Design review of the part built by this model. Coordinates are the model's own, in mm. Coordinates: 2 decimals unless noted, no trailing zeros. Loops run counter-clockwise (first coordinate to the right, second up) from the corner with the lowest first, then second, coordinate; pieces in that order, holes last. Notation, with made-up numbers: (16, 76.5) -> (37, 76.5) arc R17 cw to (37, 84.5) -> close; hole circle Ø5 at (47, -19.5). An arc over 180 degrees is marked (long way). Answer as a JSON object with one key per item and string values.
```python
from build123d import *

# Parameters (mm, degrees)
SKETCH1_W           = 698.5
SKETCH1_H           = 711.2
SKETCH1_W_2         = 203.2
SKETCH1_H_2         = 203.2
BOSS_EXTRUDE1_DEPTH = 1.5875
FILLET1_R           = 6.35
SKETCH2_R           = 2.667
SKETCH2_R_2         = 3.429
SKETCH2_R_3         = 3.175
SKETCH2_R_4         = 3.3782
SKETCH2_R_5         = 1.838164507
SKETCH2_R_6         = 1.838724473
CUT_EXTRUDE1_DEPTH  = 997.850144283
SKETCH3_W           = 50.8
SKETCH3_H           = 127
CUT_EXTRUDE2_DEPTH  = 997.850144283
SKETCH4_W           = 12.7
SKETCH4_H           = 50.8
CUT_EXTRUDE3_DEPTH  = 997.850144283
FILLET2_R           = 6.35


with BuildPart() as part:
    # Sketch1 → Boss-Extrude1 (new body)
    with BuildSketch(Plane(origin=(0, 0, 0), x_dir=(1, 0, 0), z_dir=(0, 1, 0))):
        with Locations((349.25, -355.6)):
            Rectangle(SKETCH1_W, SKETCH1_H)
        with Locations((133.35, -355.6)):
            Rectangle(SKETCH1_W_2, SKETCH1_H_2, mode=Mode.SUBTRACT)
        with Locations((565.15, -355.6)):
            Rectangle(SKETCH1_W_2, SKETCH1_H_2, mode=Mode.SUBTRACT)
    extrude(amount=BOSS_EXTRUDE1_DEPTH)

    # Fillet1
    fillet1_edges = [part.edges().sort_by_distance(p)[0] for p in [
        (31.75, 0.79375, 254),
        (31.75, 0.79375, 457.2),
        (234.95, 0.79375, 457.2),
        (234.95, 0.79375, 254),
        (463.55, 0.79375, 254),
        (463.55, 0.79375, 457.2),
        (666.75, 0.79375, 457.2),
        (666.75, 0.79375, 254),
    ]]
    fillet(fillet1_edges, radius=FILLET1_R)

    # Sketch2 → Cut-Extrude1 (cut, through all)
    with BuildSketch(Plane(origin=(0, 1.5875, 0), x_dir=(1, 0, 0), z_dir=(0, 1, 0))):
        with Locations(Location((440.3852, -407.797, 0), (0, 0, 270))):
            Circle(SKETCH2_R)
        with Locations(Location((258.1148, -407.797, 0), (0, 0, 270))):
            Circle(SKETCH2_R)
        with Locations(Location((258.1148, -303.403, 0), (0, 0, 270))):
            Circle(SKETCH2_R)
        with Locations(Location((440.3852, -303.403, 0), (0, 0, 270))):
            Circle(SKETCH2_R)
        with Locations(Location((460.248, -190.725477854, 0), (0, 0, 270))):
            Circle(SKETCH2_R_2)
        with Locations(Location((494.792, -190.725477854, 0), (0, 0, 270))):
            Circle(SKETCH2_R_2)
        with Locations(Location((460.278515752, -52.578, 0), (0, 0, 270))):
            Circle(SKETCH2_R_2)
        with Locations(Location((494.822515752, -52.578, 0), (0, 0, 270))):
            Circle(SKETCH2_R_2)
        with Locations(Location((227.307398857, -65.109713759, 0), (0, 0, 270))):
            Circle(SKETCH2_R_3)
        with Locations(Location((227.307398857, -166.709713759, 0), (0, 0, 270))):
            Circle(SKETCH2_R_3)
        with Locations(Location((93.864461583, -166.709713759, 0), (0, 0, 270))):
            Circle(SKETCH2_R_3)
        with Locations(Location((93.864461583, -65.109713759, 0), (0, 0, 270))):
            Circle(SKETCH2_R_3)
        with Locations(Location((81.164461583, -65.109713759, 0), (0, 0, 270))):
            Circle(SKETCH2_R_3)
        with Locations(Location((81.164461583, -166.709713759, 0), (0, 0, 270))):
            Circle(SKETCH2_R_3)
        with Locations(Location((238.899461934, -166.709713759, 0), (0, 0, 270))):
            Circle(SKETCH2_R_3)
        with Locations(Location((240.007398857, -65.109713759, 0), (0, 0, 270))):
            Circle(SKETCH2_R_3)
        with Locations(Location((385.445, -184.896187086, 0), (0, 0, 270))):
            Circle(SKETCH2_R_4)
        with Locations(Location((313.055, -184.896187086, 0), (0, 0, 270))):
            Circle(SKETCH2_R_4)
        with Locations(Location((593.125050357, -166.962566622, 0), (0, 0, 270))):
            Circle(SKETCH2_R_5)
        with Locations(Location((532.098143635, -166.962566622, 0), (0, 0, 270))):
            Circle(SKETCH2_R_6)
        with Locations(Location((532.083268617, -118.12580583, 0), (0, 0, 270))):
            Circle(SKETCH2_R_6)
        with Locations(Location((593.11017534, -118.12580583, 0), (0, 0, 270))):
            Circle(SKETCH2_R_5)
    extrude(amount=-CUT_EXTRUDE1_DEPTH, mode=Mode.SUBTRACT)

    # Sketch3 → Cut-Extrude2 (cut, through all)
    with BuildSketch(Plane(origin=(0, 1.5875, 0), x_dir=(1, 0, 0), z_dir=(0, 1, 0))):
        with Locations((641.35, -107.95)):
            Rectangle(SKETCH3_W, SKETCH3_H)
        with Locations((57.15, -107.95)):
            Rectangle(SKETCH3_W, SKETCH3_H)
        with Locations((57.15, -603.25)):
            Rectangle(SKETCH3_W, SKETCH3_H)
        with Locations((641.35, -603.25)):
            Rectangle(SKETCH3_W, SKETCH3_H)
    extrude(amount=-CUT_EXTRUDE2_DEPTH, mode=Mode.SUBTRACT)

    # Sketch4 → Cut-Extrude3 (cut, through all)
    with BuildSketch(Plane(origin=(0, 1.5875, 0), x_dir=(1, 0, 0), z_dir=(0, 1, 0))):
        with Locations((444.5, -98.425)):
            Rectangle(SKETCH4_W, SKETCH4_H)
        with Locations((254, -98.425)):
            Rectangle(SKETCH4_W, SKETCH4_H)
    extrude(amount=-CUT_EXTRUDE3_DEPTH, mode=Mode.SUBTRACT)

    # Fillet2
    # the kernel refuses this fillet: 6.35 mm, written as the material it adds along each edge
    with BuildSketch(Plane(origin=(438.15, 1.5875, 73.025), x_dir=(0, 0, 1), z_dir=(0, -1, 0)), Plane(origin=(450.85, 1.5875, 73.025), x_dir=(-1, 0, 0), z_dir=(0, -1, 0)), Plane(origin=(260.35, 1.5875, 73.025), x_dir=(-1, 0, 0), z_dir=(0, -1, 0)), Plane(origin=(247.65, 1.5875, 73.025), x_dir=(0, 0, 1), z_dir=(0, -1, 0)), Plane(origin=(260.35, 1.5875, 123.825), x_dir=(0, 0, -1), z_dir=(0, -1, 0)), Plane(origin=(450.85, 1.5875, 123.825), x_dir=(0, 0, -1), z_dir=(0, -1, 0)), Plane(origin=(82.55, 1.5875, 44.45), x_dir=(-1, 0, 0), z_dir=(0, -1, 0)), Plane(origin=(31.75, 1.5875, 44.45), x_dir=(0, 0, 1), z_dir=(0, -1, 0)), Plane(origin=(31.75, 1.5875, 171.45), x_dir=(1, 0, 0), z_dir=(0, -1, 0)), Plane(origin=(615.95, 1.5875, 44.45), x_dir=(0, 0, 1), z_dir=(0, -1, 0)), Plane(origin=(666.75, 1.5875, 44.45), x_dir=(-1, 0, 0), z_dir=(0, -1, 0)), Plane(origin=(31.75, 1.5875, 539.75), x_dir=(0, 0, 1), z_dir=(0, -1, 0)), Plane(origin=(31.75, 1.5875, 666.75), x_dir=(1, 0, 0), z_dir=(0, -1, 0)), Plane(origin=(615.95, 1.5875, 539.75), x_dir=(0, 0, 1), z_dir=(0, -1, 0)), Plane(origin=(666.75, 1.5875, 539.75), x_dir=(-1, 0, 0), z_dir=(0, -1, 0))) as fillet2_piece_1:
        with BuildLine():
            CenterArc((FILLET2_R, -FILLET2_R), FILLET2_R, 90, 90)
            Line((0, -FILLET2_R), (-FILLET2_R * 0.02, -FILLET2_R))
            Line((-FILLET2_R * 0.02, -FILLET2_R), (-FILLET2_R * 0.02, FILLET2_R * 0.02))
            Line((-FILLET2_R * 0.02, FILLET2_R * 0.02), (FILLET2_R, FILLET2_R * 0.02))
            Line((FILLET2_R, FILLET2_R * 0.02), (FILLET2_R, 0))
        make_face()
    extrude(amount=1.5875)
    with BuildSketch(Plane(origin=(247.65, 1.5875, 123.825), x_dir=(0, 0, -1), z_dir=(0, -1, 0)), Plane(origin=(438.15, 1.5875, 123.825), x_dir=(0, 0, -1), z_dir=(0, -1, 0)), Plane(origin=(615.95, 1.5875, 171.45), x_dir=(0, 0, -1), z_dir=(0, -1, 0)), Plane(origin=(666.75, 1.5875, 171.45), x_dir=(-1, 0, 0), z_dir=(0, -1, 0)), Plane(origin=(82.55, 1.5875, 539.75), x_dir=(0, 0, 1), z_dir=(0, -1, 0)), Plane(origin=(82.55, 1.5875, 666.75), x_dir=(-1, 0, 0), z_dir=(0, -1, 0)), Plane(origin=(615.95, 1.5875, 666.75), x_dir=(0, 0, -1), z_dir=(0, -1, 0)), Plane(origin=(666.75, 1.5875, 666.75), x_dir=(-1, 0, 0), z_dir=(0, -1, 0))) as fillet2_piece_2:
        with BuildLine():
            CenterArc((FILLET2_R, FILLET2_R), FILLET2_R, 180, 90)
            Line((0, FILLET2_R), (-FILLET2_R * 0.02, FILLET2_R))
            Line((-FILLET2_R * 0.02, FILLET2_R), (-FILLET2_R * 0.02, -FILLET2_R * 0.02))
            Line((-FILLET2_R * 0.02, -FILLET2_R * 0.02), (FILLET2_R, -FILLET2_R * 0.02))
            Line((FILLET2_R, -FILLET2_R * 0.02), (FILLET2_R, 0))
        make_face()
    extrude(amount=1.5875)
    with BuildSketch(Plane(origin=(82.55, 1.5875, 171.45), x_dir=(0, 0, -1), z_dir=(0, -1, 0))) as fillet2_piece_3:
        with BuildLine():
            CenterArc((6.35, -4.51368774), FILLET2_R, 134.698575063, 45.301424937)
            Line((0, -4.51368774), (-0.127, -4.51368774))
            Line((-0.127, -4.51368774), (-0.127, 0))
            Line((-0.127, 0), (0, 0.127))
            ThreePointArc((0, 0.127), (0.941777945, 0.127), (1.794227008, 0.090273755))
            Line((1.794227008, 0.090273755), (1.88355589, 0))
        make_face()
    extrude(amount=1.5875)


solid = part.part
```
1) Clearance check with a flat-ended pin moving along its axis: pin 1 Ø7 at (x, z) = (440.39, 407.8) entering from -Y. State where the tip first meets the part, or that it passes through.
Completed:
{"pin 1": "y = 0"}
2) Add section A-A, the plane z = 282. Give the boundary of the cut face in (x, y).
Completed:
{"outline": "(0, 0) -> (31.75, 0) -> (31.75, 1.59) -> (0, 1.59) -> close; (234.95, 0) -> (463.55, 0) -> (463.55, 1.59) -> (234.95, 1.59) -> close; (666.75, 0) -> (698.5, 0) -> (698.5, 1.59) -> (666.75, 1.59) -> close"}
3) Wall thickness on probe 1 along Z at (x, y) = (495, 0.9); probe 2 along X at (y, z) = (0.3, 575.5); probe 3 along Z at (x, y) = (656, 0.1): over which ranges is each line inside the solid? List them lowest first.
Completed:
{"probe 1": "0 to 49.15, 56 to 187.3, 194.15 to 254, 457.2 to 711.2", "probe 2": "0 to 31.75, 82.55 to 615.95, 666.75 to 698.5", "probe 3": "0 to 44.45, 171.45 to 254, 457.2 to 539.75, 666.75 to 711.2"}
4) Add section C-C, the plane y = 0.3. Count the separate pieces of the cut face and the enclosed holes in it, and give its area (3 significant figures).
Completed:
{"separate pieces": "1", "enclosed holes": "28", "area": "387,000 mm²"}
5) Add section B-B, the plane z = 567.5. Give the boundary of the cut face in (x, y), and give its area (3 significant figures).
Completed:
{"outline": "(0, 0) -> (31.75, 0) -> (31.75, 1.59) -> (0, 1.59) -> close; (82.55, 0) -> (615.95, 0) -> (615.95, 1.59) -> (82.55, 1.59) -> close; (666.75, 0) -> (698.5, 0) -> (698.5, 1.59) -> (666.75, 1.59) -> close", "area": "948 mm²"}
